Input: part model. Units: mm. Frame: model coordinates. A direction names the side the tool comes from. Coordinates: 2 decimals unless noted, no trailing zeros. Write each loop counter-clockwise with the first axis right and the second up, starting at its lowest first coordinate (ties: lowest second). Pieces come first, ordered by that corner, then holes. Notation, with made-up numbers: M -23.5,-23.5 L 33.5,-23.5 A19 ccw 33.5,-13.5 Z; hole C 27,34 d6. An arc over 180 degrees is marked long. Write each question's results on one line, items separated by ' | '. Start each with the question number.
1. Ray query, probe 1 along X at (y, z) = (-1.5, 3); probe 2 along Z at (x, y) = (-40, 2.05); probe 3 along Y at (x, z) = (7, 4.75). Return the intervals inside material, ascending.
2. Section query C-C, the plane y = 4.5. Output: boundary loops of the cut face in (x, z), and give its area (3 significant figures).
3. Set-up query: faces 4 (the flat face through (50, -3, 5)), 5 (the flat face through (-50, -3, 5)), 6 (the flat face through (50, 4, 5)), 7 (the flat face through (-47, -2, 5)), 8 (the flat face through (-50, 4, 5)). Return all of +Z, -Z, +X, -X, +Y, -Y with unobstructed straight access to the full face (end or side cutting, diameter ignored); none if empty.
4. Section query D-D, the plane y = -3.5. Output: boundary loops of the cut face in (x, z).
5. Section query B-B, the plane x = -40. Output: boundary loops of the cut face in (y, z).
6. First-contact query: pin 1 (1 mm diameter, centred on y = -3, z = 6, fed in from +X); pin 2 (2 mm diameter, centred on x = 40, z = 5, fed in from -Y); pin 3 (3 mm diameter, centred on x = 22.5, z = 3.5, fed in from -Y); pin 4 (2 mm diameter, centred on x = -50.5, z = 6.5, fed in from -Y). Flat tips, straight axial feed; report the tip coordinate or a pass-through.
7. Section query A-A, the plane z = 5. Output: boundary loops of the cut face in (x, y), and give its area (3 significant figures).
8. Pull-direction query (X, two-part tool) for faces 1 (the flat face through (52, 1, 5)), 2 (the cylindrical face through (40.99, 2.71, 4.24)), 3 (the flat face through (1, 3, 10)); classes: +X half, -X half, draft (parallel to the pull), parting line (faces both ways), or undercut.
```python
from build123d import *

# Parameters (mm, degrees)
MAINLEFT_DEPTH     = 10
SKETCH3_R          = 1.25
CUT_EXTRUDE2_DEPTH = 6.5


with BuildPart() as part:
    # Sketch1 → MainLeft (new body)
    with BuildSketch(Plane.XY):
        Polygon((-50, 5.5), (-50, 1.95), (-52, 1.95), (-52, -0.95), (-50, -0.95), (-50, -4.5), (-47, -4.5), (-47, 0), (0, 0), (0, 5.5), align=None)
    mainleft = extrude(amount=MAINLEFT_DEPTH)

    # Sketch3 → Cut-Extrude2 (cut, through all)
    with BuildSketch(Plane.XZ):
        with Locations((-40, 5)):
            Circle(SKETCH3_R)
    cut_extrude2 = extrude(amount=-CUT_EXTRUDE2_DEPTH, mode=Mode.SUBTRACT)

    # Mirror1: MainLeft, Cut-Extrude2 across plane
    add(mainleft.mirror(Plane(origin=(0, 0, 0), x_dir=(0, 0, 1), z_dir=(1, 0, 0))))
    add(cut_extrude2.mirror(Plane(origin=(0, 0, 0), x_dir=(0, 0, 1), z_dir=(1, 0, 0))), mode=Mode.SUBTRACT)


solid = part.part
```
Answer:
1) probe 1: -50 to -47, 47 to 50 | probe 2: 0 to 3.75, 6.25 to 10 | probe 3: 0 to 5.5
2) outline: M -50,0 L 50,0 L 50,10 L -50,10 Z; hole C -40,5 d2.5; hole C 40,5 d2.5 | area: 990 mm^2
3) face 4: +Z, -Z, +X, -Y | face 5: +Z, -Z, -X, -Y | face 6: +Z, -Z, +X, +Y | face 7: +Z, -Z, -Y | face 8: +Z, -Z, -X, +Y
4) outline: M -50,0 L -47,0 L -47,10 L -50,10 Z; M 47,0 L 50,0 L 50,10 L 47,10 Z
5) outline: M 0,0 L 5.5,0 L 5.5,3.75 L 0,3.75 Z; M 0,6.25 L 5.5,6.25 L 5.5,10 L 0,10 Z
6) pin 1: x = 50 | pin 2: through | pin 3: y = 0 | pin 4: y = -4.5
7) outline: M -52,-0.95 L -50,-0.95 L -50,-4.5 L -47,-4.5 L -47,0 L -41.25,0 L -41.25,5.5 L -50,5.5 L -50,1.95 L -52,1.95 Z; M -38.75,0 L 38.75,0 L 38.75,5.5 L -38.75,5.5 Z; M 41.25,0 L 47,0 L 47,-4.5 L 50,-4.5 L 50,-0.95 L 52,-0.95 L 52,1.95 L 50,1.95 L 50,5.5 L 41.25,5.5 Z | area: 561 mm^2
8) face 1: +X half | face 2: undercut | face 3: draft
